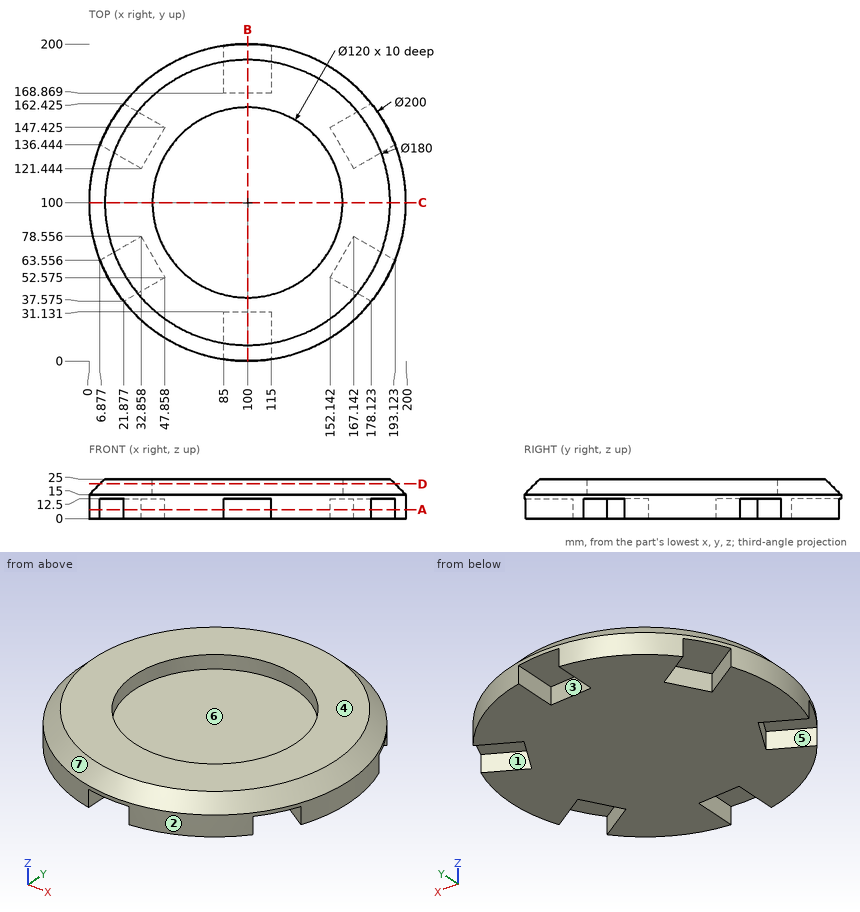
Print and shaded views of the part. All mm, measured from the part's lowest x, y and z. A direction names the side the tool comes from. Give positions to 0.01 mm unless a question says otherwise; leave off trailing zeros. Order: outer loops, then holes, each group sorted by start corner. A loop starts at its lowest first (then second) coordinate and runs counter-clockwise, first axis right, second up. Notation, with made-up numbers: (86.25, 78) -> (97.25, 78) arc R16 cw to (97.25, 89) -> close; hole circle Ø6 at (49.5, 43). An arc over 180 degrees is marked (long way). Use CSV: the item, a comma, the result in double quotes.
1. Band-saw the part on C-C, the plane y = 100. Give the cut face in (x, z), then the cut area to 3 significant figures.
Outcome:
outline,"(0, 0) -> (200, 0) -> (200, 15) -> (190, 25) -> (160, 25) -> (160, 15) -> (40, 15) -> (40, 25) -> (10, 25) -> (0, 15) -> close"
area,"3,700 mm²"
2. Drop flat-ended pins along their axis: pin 1 (6 mm diameter, centred on x = 98, z = 4, fed in from -Y); pin 2 (10 mm diameter, centred on y = 12, z = 7.5, fed in from +X) (1 decimal); pin 3 (6 mm diameter, centred on y = 174, z = 8, fed in from -X). Give the stop position or say it passes through.
Outcome:
pin 1,"y = 31.13"
pin 2,"x = 155.8"
pin 3,"x = 29.58"
3. 3-axis set-ups, long thin cutter, end or side, ignore diameter. For the marked faces 1, 2 and 3: which of +Z, -Z, +X, -X, +Y, -Y reach the whole face in a straight line?
Outcome:
face 1,"-Z"
face 2,"+Z, -Z"
face 3,"-Z, +Y"
4. Drill centre lines: line 1 along Y through (x, z) = (177, 4.5) (1 decimal); line 2 along Z through (x, y) = (114, 145); line 3 along X through (y, z) = (19.5, 7) (1 decimal). Where is each one in solid material? Low to high. Write a range as from..to.
Outcome:
line 1,"36.2..38.2, 72.9..127.1, 161.8..163.8"
line 2,"0..15"
line 3,"40.7..85, 115..159.3"
5. Band-saw the part on D-D, the plane z = 22. Give the cut face in (x, y).
Outcome:
outline,"circle Ø186 at (100, 100); hole circle Ø120 at (100, 100)"
6. Band-saw the part on B-B, the plane x = 100. Give the cut face in (y, z), then the cut area to 3 significant figures.
Outcome:
outline,"(0, 12.5) -> (31.13, 12.5) -> (31.13, 0) -> (168.87, 0) -> (168.87, 12.5) -> (200, 12.5) -> (200, 15) -> (190, 25) -> (160, 25) -> (160, 15) -> (40, 15) -> (40, 25) -> (10, 25) -> (0, 15) -> close"
area,"2,920 mm²"
7. Band-saw the part on A-A, the plane z = 5.75. Give the cut face in (x, y) (1 decimal), then the cut area to 3 significant figures.
Outcome:
outline,"(6.9, 63.6) -> (32.9, 78.6) -> (47.9, 52.6) -> (21.9, 37.6) arc R100 ccw to (85, 1.1) -> (85, 31.1) -> (115, 31.1) -> (115, 1.1) arc R100 ccw to (178.1, 37.6) -> (152.1, 52.6) -> (167.1, 78.6) -> (193.1, 63.6) arc R100 ccw to (193.1, 136.4) -> (167.1, 121.4) -> (152.1, 147.4) -> (178.1, 162.4) arc R100 ccw to (115, 198.9) -> (115, 168.9) -> (85, 168.9) -> (85, 198.9) arc R100 ccw to (21.9, 162.4) -> (47.9, 147.4) -> (32.9, 121.4) -> (6.9, 136.4) arc R100 ccw to start"
area,"25,900 mm²"
8. Mould opens along X. For the marked faces 4, 5, 6 and 7 say: +X half, -X half, draft (parallel to the pull), parting line (faces both ways), or undercut.
Outcome:
face 4,"draft"
face 5,"-X half"
face 6,"undercut"
face 7,"parting line"
